Read the model definition and answer for the solid it produces. Units are mm, in the model's axes. A direction names the side the tool comes from. Coordinates: 2 decimals unless noted, no trailing zeros. Loops run counter-clockwise (first coordinate to the right, second up) from the corner with the lowest first, then second, coordinate; pieces in that order, holes last. Notation, with made-up numbers: (-24.75, 14) - (-0.75, 14) arc R22 cw to (-0.75, 44) - close; hole circle Ø2 at (10, -1). An arc over 180 degrees is marked (long way). One line per question, with ' | ' between items. Start each with the question number.
```python
from build123d import *

# Parameters (mm, degrees)
SKETCH1_W                          = 25.4
SKETCH1_H                          = 76.2
EXTRUDE1_DEPTH                     = 20.447
SKETCH60_W                         = 25.4
SKETCH60_H                         = 63.5
EXTRUDE6_DEPTH                     = 63.5
SKETCH69_W                         = 63.5
SKETCH69_H                         = 63.5
SKETCH69_R                         = 22.225
CUT_EXTRUDE23_DEPTH                = 4.953
SKETCH71_R                         = 9.525
CUT_EXTRUDE24_DEPTH                = 24.778013047
SKETCH80_W                         = 20.447
SKETCH80_H                         = 76.2
EXTRUDE11_DEPTH                    = 6.35
SKETCH76_W                         = 25.4
SKETCH76_H                         = 76.2
EXTRUDE9_DEPTH                     = 25.4
SKETCH79_W                         = 50.8
SKETCH79_H                         = 6.35
EXTRUDE10_DEPTH                    = 46.847
SKETCH84_W                         = 60.325
SKETCH84_H                         = 25.4
EXTRUDE14_DEPTH                    = 15.24
EXTRUDE14_DEPTH_BACK               = 12.7
EXTRUDE15_DEPTH                    = 1.524
CBORE_FOR_1_8_PRESS_PIN_AT_2_COUNT = 2
CBORE_FOR_1_8_PRESS_PIN_AT_2_PITCH = 38.1
CHAMFER5_SIZE                      = 9.525
FILLET6_R                          = 12.7
CHAMFER3_SIZE                      = 12.7
FILLET7_R                          = 0.254
CHAMFER4_SIZE                      = 0.762
FILLET4_R                          = 2.54
FILLET5_R                          = 0.635


with BuildPart() as part:
    # Sketch1 → Extrude1 (new body)
    with BuildSketch(Plane.XY):
        with Locations((12.7, 0)):
            Rectangle(SKETCH1_W, SKETCH1_H)
    extrude(amount=EXTRUDE1_DEPTH)

    # Sketch60 → Extrude6 (add)
    with BuildSketch(Plane.ZY):
        with Locations((7.747, 0)):
            Rectangle(SKETCH60_W, SKETCH60_H)
    extrude(amount=EXTRUDE6_DEPTH)

    # Sketch64 → Cut-Revolve1 (revolve, cut)
    with BuildSketch(Plane(origin=(0, 0, 0), x_dir=(-1, 0, 0), z_dir=(0, 1, 0)), mode=Mode.PRIVATE) as cut_revolve1_sk:
        with BuildLine():
            Line((9.525, -4.953), (9.525, 0.012163278))
            ThreePointArc((9.525, 0.012163278), (14.839678796, -1.926851671), (20.32, -3.331013047))
            Line((20.32, -3.331013047), (31.75, -3.331013047))
            Line((31.75, -3.331013047), (31.75, -4.953))
            Line((31.75, -4.953), (9.525, -4.953))
        make_face()
        with BuildLine():
            Line((31.75, 20.447), (11.43, 20.447))
            ThreePointArc((11.43, 20.447), (21.174424434, 16.073156441), (31.75, 14.575986953))
            Line((31.75, 14.575986953), (31.75, 20.447))
        make_face()
    revolve(cut_revolve1_sk.sketch.rotate(Axis((-31.75, 0, 14.575986953), (0, 0, 1)), 180), axis=Axis((-31.75, 0, 14.575986953), (0, 0, 1)), mode=Mode.SUBTRACT)  # turned: the seam where the file's is

    # Sketch69 → Cut-Extrude23 (cut)
    with BuildSketch(Plane(origin=(0, 0, -4.953), x_dir=(-1, 0, 0), z_dir=(0, 0, -1))):
        with Locations((31.75, 0)):
            Rectangle(SKETCH69_W, SKETCH69_H)
        with Locations((31.75, 0)):
            Circle(SKETCH69_R, mode=Mode.SUBTRACT)
    extrude(amount=-CUT_EXTRUDE23_DEPTH, mode=Mode.SUBTRACT)

    # Sketch71 → Cut-Extrude24 (cut, through all)
    with BuildSketch(Plane.XY.offset(20.447)):
        with Locations((-31.75, 0)):
            Circle(SKETCH71_R)
    extrude(amount=-CUT_EXTRUDE24_DEPTH, mode=Mode.SUBTRACT)

    # Sketch80 → Extrude11 (add)
    with BuildSketch(Plane(origin=(25.4, 0, 0), x_dir=(0, 0, -1), z_dir=(1, 0, 0))):
        with Locations((-10.2235, 0)):
            Rectangle(SKETCH80_W, SKETCH80_H)
    extrude(amount=EXTRUDE11_DEPTH)

    # Sketch76 → Extrude9 (add)
    with BuildSketch(Plane(origin=(0, 0, 0), x_dir=(-1, 0, 0), z_dir=(0, 0, -1))):
        with Locations((-19.05, 0)):
            Rectangle(SKETCH76_W, SKETCH76_H)
    extrude(amount=EXTRUDE9_DEPTH)

    # Sketch79 → Extrude10 (cut, through all)
    with BuildSketch(Plane.XY.offset(20.447)):
        with Locations((6.35, -34.925)):
            Rectangle(SKETCH79_W, SKETCH79_H)
        with Locations((6.35, 34.925)):
            Rectangle(SKETCH79_W, SKETCH79_H)
    extrude(amount=-EXTRUDE10_DEPTH, mode=Mode.SUBTRACT)

    # Sketch84 → Extrude14 (add, two sides)
    with BuildSketch(Plane(origin=(0, 31.75, 0), x_dir=(1, 0, 0), z_dir=(0, 1, 0))) as extrude14_sk:
        with Locations((36.5125, 12.7)):
            Rectangle(SKETCH84_W, SKETCH84_H)
    extrude(amount=EXTRUDE14_DEPTH)
    extrude(extrude14_sk.sketch, amount=-EXTRUDE14_DEPTH_BACK)

    # Sketch85 → CBORE for 1_4 Socket Head Cap Screw1 (revolve, cut)
    with BuildSketch(Plane(origin=(19.05, -31.75, -10.16), x_dir=(0, 0, -1), z_dir=(1, 0, 0))):
        Polygon((0, 0), (0, 78.74), (4.20624, 78.74), (3.57124, 78.105), (3.57124, 50.8), (6.35, 50.8), (6.35, 0.762), (7.112, 0), align=None)
    revolve(axis=Axis((19.05, -38.1, -10.16), (0, 1, 0)), mode=Mode.SUBTRACT)

    # Sketch87 → 1_4 Clearance Hole2 (revolve, cut)
    with BuildSketch(Plane(origin=(57.15, 19.05, -10.16), x_dir=(0, 0, -1), z_dir=(1, 0, 0))):
        Polygon((0, 0), (0, 27.94), (4.20624, 27.94), (3.57124, 27.305), (3.57124, 0), align=None)
    revolve(axis=Axis((57.15, 12.7, -10.16), (0, 1, 0)), mode=Mode.SUBTRACT)

    # Sketch89 → Extrude15 (cut)
    with BuildSketch(Plane(origin=(0, 46.99, 0), x_dir=(1, 0, 0), z_dir=(0, 1, 0))):
        Polygon((6.35, 3.81), (66.675, 3.81), (66.675, 16.51), (63.5, 16.51), (63.5, 25.4), (56.896, 25.4), (56.896, 16.51), (25.146, 16.51), (25.146, 25.4), (18.542, 25.4), (18.542, 16.51), (6.35, 16.51), align=None)
    extrude(amount=-EXTRUDE15_DEPTH, mode=Mode.SUBTRACT)

    # Sketch90 → CBORE for 1_8_ Press Pin (revolve, cut)
    with BuildSketch(Plane(origin=(22.225, 45.466, -20.955), x_dir=(0, 0, 1), z_dir=(1, 0, 0))):
        Polygon((0, 0), (0, 7.303866233), (1.5875, 6.35), (1.5875, 1.524), (1.6002, 1.524), (1.6002, 0.3048), (1.905, 0), align=None)
    cbore_for_1_8_press_pin = revolve(axis=Axis((22.225, 51.816, -20.955), (0, -1, 0)), mode=Mode.SUBTRACT)

    # CBORE for 1_8_ Press Pin at 2: CBORE for 1_8_ Press Pin ×2
    with Locations(*[(i * CBORE_FOR_1_8_PRESS_PIN_AT_2_PITCH, 0, 0) for i in range(1, CBORE_FOR_1_8_PRESS_PIN_AT_2_COUNT)]):
        add(cbore_for_1_8_press_pin, mode=Mode.SUBTRACT)

    # Chamfer5
    chamfer5_edges = [part.edges().sort_by_distance(p)[0] for p in [
        (6.35, 7.62, -25.4),
    ]]
    chamfer(chamfer5_edges, length=CHAMFER5_SIZE)

    # Fillet6
    fillet6_edges = [part.edges().sort_by_distance(p)[0] for p in [
        (31.75, 19.05, -12.7),
    ]]
    fillet(fillet6_edges, radius=FILLET6_R)

    # Chamfer3
    chamfer3_edges = [part.edges().sort_by_distance(p)[0] for p in [
        (-63.5, 31.75, 10.2235),
        (-63.5, -31.75, 10.2235),
        (31.75, 31.75, 10.2235),
    ]]
    chamfer(chamfer3_edges, length=CHAMFER3_SIZE)

    # Fillet7
    fillet7_edges = [part.edges().sort_by_distance(p)[0] for p in [
        (6.35, 0, 0),
    ]]
    fillet(fillet7_edges, radius=FILLET7_R)

    # Chamfer4
    chamfer4_edges = [part.edges().sort_by_distance(p)[0] for p in [
        (23.8125, -31.75, -25.4),
        (-9.525, -31.75, 20.447),
        (31.75, -6.35, 20.447),
        (31.75, -31.75, -2.4765),
        (-22.352, -31.75, 0),
        (6.275605122, -31.75, -0.074394878),
        (6.35, -31.75, -8.0645),
        (-57.15, 25.4, 20.447),
        (-57.15, 25.4, 0),
        (-57.15, -25.4, 0),
        (-57.15, -25.4, 20.447),
        (-63.5, 0, 20.447),
        (-63.5, 0, 0),
        (11.1125, -31.75, -20.6375),
    ]]
    chamfer(chamfer4_edges, length=CHAMFER4_SIZE)

    # Fillet4
    fillet4_edges = [part.edges().sort_by_distance(p)[0] for p in [
        (-20.32, 0, -3.331013047),
    ]]
    fillet(fillet4_edges, radius=FILLET4_R)

    # Fillet5
    fillet5_edges = [part.edges().sort_by_distance(p)[0] for p in [
        (-11.43, 0, 20.447),
    ]]
    fillet(fillet5_edges, radius=FILLET5_R)


solid = part.part
```
1) Given pin 1 Ø16.5 at (x, z) = (-22.5, 12) entering from +Y; pin 2 Ø0.8 at (y, z) = (46, -20.5) entering from -X (3 decimals); pin 3 Ø2.5 at (x, z) = (60.325, -20.955) entering from +Y, each flat-ended and moving along its own axis, determine where each tip first touches the part or whether it passes through.
2) The part is cut by section B-B on y = 0. Count the separate pieces of the cut face and the enclosed holes in it, and give its area (3 significant figures).
3) The part is cut by section C-C on x = 38.5. Write down the section's boundary in (y, z).
4) Find the intervals of material crossed by line 1 along Y through (x, z) = (-31.5, 12); line 2 along Z through (x, y) = (57.15, 32.75); line 3 along X through (y, z) = (24.5, -2) (3 decimals), in increasing order. Write a range as from..to.
5) Which of the six approach directions +Z, -Z, +X, -X, +Y, -Y give full straight-line access (tool end or side, diameter ignored) to faces 1 (the flat face through (53, 19.05, -13)), 2 (the flat face through (-14, 14, 0)), 3 (the cylindrical face through (24.684, -6.319, -13.09)), 4 (the flat face through (11.31, -31.36, -20.31)), 5 (the flat face through (25.5, 25.3, 10.4))?
6) The part is cut by section A-A on z = -10.16. Write down the section's boundary in (x, y) (3 decimals), and give its area (3 significant figures).
Answer below:
1) pin 1: y = 31.75 | pin 2: x = 10.575 | pin 3: y = 38.91
2) separate pieces: 2 | enclosed holes: 1 | area: 2,030 mm2
3) outline: (17.57, -25.4) - (46.99, -25.4) - (46.99, -16.51) - (45.47, -16.51) - (45.47, -3.81) - (46.99, -3.81) - (46.99, 0) - (17.57, 0) - close
4) line 1: -31.75..-9.52, 9.52..31.75 | line 2: -25.4..-13.73, -6.59..0 | line 3: 6.35..66.675
5) face 1: +Z, -Z, +X, -Y | face 2: -Z | face 3: -Y | face 4: -Z, -X, -Y | face 5: +Z, +X, +Y
6) outline: (6.35, -30.988) - (7.112, -31.75) - (11.938, -31.75) - (12.7, -30.988) - (12.7, 19.05) - (15.479, 19.05) - (15.479, 45.466) - (6.35, 45.466) - close; (22.621, 19.05) - (25.4, 19.05) - (25.4, -30.988) - (26.162, -31.75) - (30.988, -31.75) - (31.75, -30.988) - (31.75, 6.35) arc R12.7 cw to (44.45, 19.05) - (53.579, 19.05) - (53.579, 45.466) - (22.621, 45.466) - close; (60.721, 19.05) - (66.675, 19.05) - (66.675, 45.466) - (60.721, 45.466) - close | area: 1,890 mm2
